```python
from build123d import *

# Parameters (mm, degrees)
CORTE_EXTERIOR_R        = 1.05
CORTE_EXTERIOR_R_2      = 3.5
SALIENTE_EXTRUIR1_DEPTH = 3
CORTAR_EXTRUIR1_DEPTH   = 0.1


with BuildPart() as part:
    # Corte exterior → Saliente-Extruir1 (new body)
    with BuildSketch(Plane.XY):
        Polygon((28.7, -4.2), (23.7, -4.2), (23.7, -1.2), (18.7, -1.2), (18.7, 9.8), (18.7, 31.8), (23.7, 31.8), (23.7, 34.8), (28.7, 34.8), (28.7, 31.8), (33.7, 31.8), (33.7, 15.8), (33.7, -1.2), (28.7, -1.2), align=None)
        with Locations((26.2, 25.972229454)):
            Circle(CORTE_EXTERIOR_R, mode=Mode.SUBTRACT)
        with Locations((26.2, 4.627770547)):
            Circle(CORTE_EXTERIOR_R, mode=Mode.SUBTRACT)
        with Locations((26.2, 15.3)):
            Circle(CORTE_EXTERIOR_R_2, mode=Mode.SUBTRACT)
    extrude(amount=SALIENTE_EXTRUIR1_DEPTH)

    # Grabado Superficie → Cortar-Extruir1 (cut)
    with BuildSketch(Plane.XY):
        with BuildLine():
            Line((22.930825792, 16.55), (24.2, 29.3))
            ThreePointArc((24.2, 29.3), (26.101579532, 31.297576885), (28.190313411, 29.496602453))
            Line((28.190313411, 29.496602453), (29.469174208, 16.55))
            ThreePointArc((29.469174208, 16.55), (26.2, 18.8), (22.930825792, 16.55))
        make_face()
        with BuildLine():
            Line((29.469174208, 14.05), (28.2, 1))
            ThreePointArc((28.2, 1), (26.2, -1), (24.2, 1))
            Line((24.2, 1), (22.930825792, 14.05))
            ThreePointArc((22.930825792, 14.05), (26.2, 11.8), (29.469174208, 14.05))
        make_face()
    extrude(amount=CORTAR_EXTRUIR1_DEPTH, mode=Mode.SUBTRACT)


solid = part.part
```
Could you check a few things on this model? Use its own coordinates, in mm. A direction names the side the tool comes from. Coordinates: 2 decimals unless noted, no trailing zeros. Loops run counter-clockwise (first coordinate to the right, second up) from the corner with the lowest first, then second, coordinate; pieces in that order, holes last. Notation, with made-up numbers: M -31,63 L 24,63 A21 ccw 24,70 Z; hole C 59.5,69.5 d10. An arc over 180 degrees is marked long. Put each result on its own line as item: value. Start each with the question number.
(1) For faces 4 (the face through (23.7, 33, 1)), 5 (the face through (21, -1.2, 1)), 6 (the face through (26, 24, 0.1)), 7 (the face through (28.7, -3, 1)), which set-ups out of +Z, -Z, +X, -X, +Y, -Y let a thin tool reach every point of the face, with its end or its side?
(2) Thinking about a two-plate mould opening in Y: for faces 1 (the face through (31, -1.2, 1)), 2 (the face through (26.063, 27.013, 1.53)), 3 (the face through (21, 31.8, 1)), which applies, pulls with the +Y half, pulls with the -Y half, needs draft (parallel to the pull), parting line crosses it, or undercut?
(3) Will these pins go through, and if not, where does the flat tip stop? P1, Ø1.5, axis at y = -3, z = 2, coming from the +X side; P2, Ø1, axis at x = 29.5, z = 1, coming from the -Y side; P3, Ø5.5, axis at x = 26.2, y = 15.3, coming from the -Z side; P4, Ø2, axis at x = 25.5, y = 23, coming from the -Z side.
(4) Suppose I cut it at B-B on y = 15.3. Please give me the cut outline in (x, z).
(5) I need wall thicknesses on line 1 (Y direction, x = 26.25, z = 2.15); line 2 (X direction, y = 15.3, z = 1.35); line 3 (Y direction, x = 26.5, z = 2.75). Which ranges of each line are inside material? Lowest first, please. Write a range as from..to.
(6) Suppose I cut it at A-A on x = 26.2. Please give me the cut outline in (y, z).
(7) Suppose I cut it at C-C on z = 2.15. Please give me the cut outline in (x, y).
Solutions:
1. face 4: +Z, -Z, -X, +Y
1. face 5: +Z, -Z, -X, -Y
1. face 6: -Z
1. face 7: +Z, -Z, +X, -Y
2. face 1: pulls with the -Y half
2. face 2: undercut
2. face 3: pulls with the +Y half
3. P1: stops at x = 28.7
3. P2: stops at y = -1.2
3. P3: passes through
3. P4: stops at z = 0.1
4. outline: M 18.7,0 L 22.7,0 L 22.7,3 L 18.7,3 Z; M 29.7,0 L 33.7,0 L 33.7,3 L 29.7,3 Z
5. line 1: y = -4.2..3.58, 5.68..11.8, 18.8..24.92, 27.02..34.8
5. line 2: x = 18.7..22.7, 29.7..33.7
5. line 3: y = -4.2..3.62, 5.63..11.81, 18.79..24.97, 26.98..34.8
6. outline: M -4.2,0 L -1,0 L -1,0.1 L 3.58,0.1 L 3.58,3 L -4.2,3 Z; M 5.68,0.1 L 11.8,0.1 L 11.8,3 L 5.68,3 Z; M 18.8,0.1 L 24.92,0.1 L 24.92,3 L 18.8,3 Z; M 27.02,0.1 L 31.3,0.1 L 31.3,0 L 34.8,0 L 34.8,3 L 27.02,3 Z
7. outline: M 18.7,-1.2 L 23.7,-1.2 L 23.7,-4.2 L 28.7,-4.2 L 28.7,-1.2 L 33.7,-1.2 L 33.7,31.8 L 28.7,31.8 L 28.7,34.8 L 23.7,34.8 L 23.7,31.8 L 18.7,31.8 Z; hole C 26.2,15.3 d7; hole C 26.2,4.63 d2.1; hole C 26.2,25.97 d2.1
